from build123d import *

# Parameters (mm, degrees)
FILLET1_R = 2


with BuildPart() as part:
    # Sketch2 → Revolve1 (revolve)
    with BuildSketch(Plane.XY, mode=Mode.PRIVATE) as revolve1_sk:
        Polygon((-20, 10), (20, 10), (20, 12), (1.25, 14.635140651), (1.25, 36), (14.5, 36), (14.5, 40), (-14.5, 40), (-14.5, 36), (-1.25, 36), (-1.25, 14.635140651), (-20, 12), align=None)
    revolve(revolve1_sk.sketch.rotate(Axis((0, 0, 0), (1, 0, 0)), 90), axis=Axis((0, 0, 0), (1, 0, 0)))

    # Fillet1
    fillet1_edges = [part.edges().sort_by_distance(p)[0] for p in [
        (14.5, 0, -40),
        (-14.5, 0, -40),
        (-14.5, 0, -36),
        (14.5, 0, -36),
    ]]
    fillet(fillet1_edges, radius=FILLET1_R - 0.0001)  # a hair under: the kernel refuses the full size


solid = part.part
Could you check a few things on this model? Use its own coordinates, in mm. A direction names the side the tool comes from. Give positions to 0.01 mm unless a question says otherwise; leave off trailing zeros. Order: outer loops, then holes, each group sorted by start corner. A loop starts at its lowest first (then second) coordinate and runs counter-clockwise, first axis right, second up.
Item 1: If we section it at C-C, the plane x = 5: Write out the boundary of the cut face in (y, z).
Item 2: I need wall thicknesses on line 1 (Y direction, x = -6, z = 0); line 2 (Z direction, x = 4, y = -11.5); line 3 (Y direction, x = 9, z = 0). Which ranges of each line are inside material? Lowest first, please.
Item 3: I'm going to push flat-ended pins straight in: pin 1 (3 mm diameter, centred on y = -26.5, z = 25.5, fed in from -X); pin 2 (12 mm diameter, centred on x = 7.5, y = -19, fed in from +Z); pin 3 (4 mm diameter, centred on x = -1.5, y = 25, fed in from +Z). Where does each tip first touch, or does it pass through?
Item 4: For faces 5 (the face through (6.954, -24.331, -26.533)), 6 (the face through (0, 0, -10)), 7 (the face through (-1.25, 15, -1)), which set-ups out of +Z, -Z, +X, -X, +Y, -Y let a thin tool reach every point of the face, with its end or its side?
Item 5: If we mould it in two halves opening along Y, with no side actions, what happens to faces 1 (the face through (-6.796, -24.331, -26.533)), 2 (the face through (-20, -9, -5)), 3 (the face through (-0.18, -1.76, -39.96)), 4 (the face through (1.25, 15, 1))? For each: pulls with the +Y half, pulls with the -Y half, needs draft (parallel to the pull), parting line crosses it, or undercut.
Values:
1. outline: circle Ø80 at (0, 0); circle Ø28.22 at (0, 0); hole circle Ø72 at (0, 0); hole circle Ø20 at (0, 0)
2. line 1: y = -40 to -36, -13.97 to -10, 10 to 13.97, 36 to 40
2. line 2: z = -38.31 to -34.11, -8.41 to 8.41, 34.11 to 38.31
2. line 3: y = -40 to -36, -13.55 to -10, 10 to 13.55, 36 to 40
3. pin 1: stops at x = -14.5
3. pin 2: stops at z = 37.83
3. pin 3: stops at z = 32.73
4. face 5: +X
4. face 6: +X, -X
4. face 7: -X
5. face 1: undercut
5. face 2: needs draft
5. face 3: parting line crosses it
5. face 4: undercut
